Geometry: final body of the model. Coordinates: model frame, mm. Face numbers are marked on the shaded views. A direction names the side the tool comes from. Round coordinates to 2 decimals unless told otherwise and drop trailing zeros. Write each loop counter-clockwise with the first axis right and the second up, starting at its lowest first coordinate (ties: lowest second). Pieces come first, ordered by that corner, then holes. Notation, with made-up numbers: M 9.25,36.5 L 16.25,36.5 A27 ccw 16.25,69.5 Z; hole C 9,44.5 d5. An arc over 180 degrees is marked long. Use one line per item in the form item = value. Start each with the question number.
Item 1: Pull-direction query (Z, two-part tool) for the marked faces 4, 5 and 6; classes: pulls with the +Z half, pulls with the -Z half, needs draft (parallel to the pull), parting line crosses it, or undercut.
Item 2: Ray query, probe 1 along Y at (x, z) = (5.5, -7); probe 2 along Y at (x, z) = (-6.5, -25.5); probe 3 along Y at (x, z) = (-12, -20.5). Return the intervals inside material, ascending.
Item 3: Pin query (flat end, axial travel): pin 1 Ø4 at (x, y) = (1, 54) entering from -Z; pin 2 Ø15.5 at (y, z) = (41.5, 23) entering from -X; pin 3 Ø2.5 at (x, z) = (-25.5, 9.5) entering from +Y; pin 4 Ø12 at (x, z) = (-10.5, 21) entering from -Y. Return the tip coordinate at first contact, or that it passes through.
Item 4: Section query C-C (y = 65). Return loops of the section in (x, z), and give its area (3 significant figures).
Item 5: Reachability of the marked faces 1, 2 and 3 from +Z, -Z, +X, -X, +Y, -Y: full face, straight path, thin tool, end or side. Return the list, or none.
Item 6: Section query A-A (x = 0). Return loops of the section in (y, z).
Item 7: Section query B-B (y = 31.5). Return loops of the section in (x, z).
from build123d import *

# Parameters (mm, degrees)
CUT_EXTRUDE1_DEPTH = 14


with BuildPart() as part:
    # Sketch1 → Revolve1 (revolve)
    with BuildSketch(Plane.XY, mode=Mode.PRIVATE) as revolve1_sk:
        Polygon((0, 0), (0, 71), (4, 71), (4, 50), (15.241746612, 50), (30, 35.241746612), (30, 10.816092816), (25, 10.816092816), (25, 0), align=None)
        Polygon((4, 46.870301593), (15.276378104, 46.870301593), (26.904933085, 35.241746612), (4, 35.241746612), align=None, mode=Mode.SUBTRACT)
    revolve(revolve1_sk.sketch.rotate(Axis((0, 0, 0), (0, 1, 0)), 90), axis=Axis((0, 0, 0), (0, 1, 0)))

    # Sketch2 → Cut-Extrude1 (cut)
    with BuildSketch(Plane(origin=(0, 50, 0), x_dir=(1, 0, 0), z_dir=(0, 1, 0))):
        with BuildLine():
            Line((4, -13.71219958), (4, -33.089481043))
            Line((4, -33.089481043), (-4, -33.089481043))
            Line((-4, -33.089481043), (-4, -13.71219958))
            ThreePointArc((-4, -13.71219958), (0, -9.71219958), (4, -13.71219958))
        make_face()
        with BuildLine():
            Line((-30.23389859, -14.029438043), (-32.706034545, -6.420985912))
            Line((-32.706034545, -6.420985912), (-14.277144741, -0.433076635))
            ThreePointArc((-14.277144741, -0.433076635), (-9.236850698, -3.001234723), (-11.805008786, -8.041528766))
            Line((-11.805008786, -8.041528766), (-30.23389859, -14.029438043))
        make_face()
        with BuildLine():
            Line((-22.685576941, 24.41881149), (-16.213440986, 29.121093508))
            Line((-16.213440986, 29.121093508), (-4.823760712, 13.4445435))
            ThreePointArc((-4.823760712, 13.4445435), (-5.708687681, 7.857334513), (-11.295896667, 8.742261481))
            Line((-11.295896667, 8.742261481), (-22.685576941, 24.41881149))
        make_face()
        with BuildLine():
            Line((16.213440986, 29.121093508), (22.685576941, 24.41881149))
            Line((22.685576941, 24.41881149), (11.295896667, 8.742261481))
            ThreePointArc((11.295896667, 8.742261481), (5.708687681, 7.857334513), (4.823760712, 13.4445435))
            Line((4.823760712, 13.4445435), (16.213440986, 29.121093508))
        make_face()
        with BuildLine():
            Line((32.706034545, -6.420985912), (30.23389859, -14.029438043))
            Line((30.23389859, -14.029438043), (11.805008786, -8.041528766))
            ThreePointArc((11.805008786, -8.041528766), (9.236850698, -3.001234723), (14.277144741, -0.433076635))
            Line((14.277144741, -0.433076635), (32.706034545, -6.420985912))
        make_face()
    extrude(amount=-CUT_EXTRUDE1_DEPTH, mode=Mode.SUBTRACT)


solid = part.part
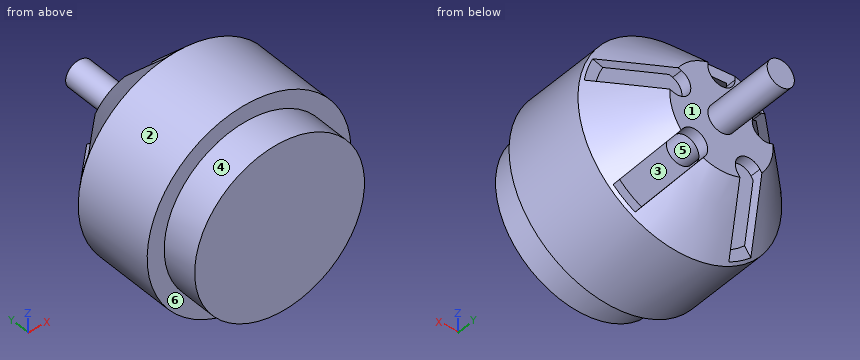
Working result:
q1.face_4 = parting line crosses it
q1.face_5 = undercut
q1.face_6 = needs draft
q2.probe_1 = 0 to 35.24, 46.87 to 50
q2.probe_2 = 10.82 to 35.24, 35.83 to 38.93
q2.probe_3 = 0 to 35.24
q3.pin_1 = -4
q3.pin_2 = -23.67
q3.pin_3 = 36
q3.pin_4 = 0
q4.outline = C 0,0 d8
q4.area = 50.3 mm²
q5.face_1 = +Y
q5.face_2 = +Y, -Y
q5.face_3 = none
q6.outline = M 0,-25 L 10.82,-25 L 10.82,-30 L 35.24,-30 L 50,-15.24 L 50,-4 L 71,-4 L 71,4 L 50,4 L 50,9.71 L 46.87,9.71 L 46.87,4 L 35.24,4 L 35.24,26.9 L 36,26.15 L 36,29.24 L 35.24,30 L 10.82,30 L 10.82,25 L 0,25 Z; hole M 35.24,-26.9 L 46.87,-15.28 L 46.87,-4 L 35.24,-4 Z
q7.outline = C 0,0 d60
